```python
from build123d import *

# Parameters (mm, degrees)
BOSS_EXTRUDE1_DEPTH         = 6.35
FILLET1_R                   = 6.35
FILLET2_R                   = 1.5875
F_1_4_0_25_DIAMETER_HOLE1_D = 6.35


with BuildPart() as part:
    # Sketch2 → Boss-Extrude1 (new body)
    with BuildSketch(Plane.XY):
        with BuildLine():
            Line((-47.625, -279.4), (-26.924, -279.4))
            Line((-26.924, -279.4), (-26.924, -254))
            ThreePointArc((-26.924, -254), (0, -227.076), (26.924, -254))
            Line((26.924, -254), (26.924, -279.4))
            Line((26.924, -279.4), (47.625, -279.4))
            Line((47.625, -279.4), (47.625, 12.7))
            Line((47.625, 12.7), (26.924, 12.7))
            Line((26.924, 12.7), (26.924, -44.45))
            ThreePointArc((26.924, -44.45), (0, -71.374), (-26.924, -44.45))
            Line((-26.924, -44.45), (-26.924, 12.7))
            Line((-26.924, 12.7), (-47.625, 12.7))
            Line((-47.625, 12.7), (-47.625, -279.4))
        make_face()
    extrude(amount=BOSS_EXTRUDE1_DEPTH)

    # Fillet1
    fillet1_edges = [part.edges().sort_by_distance(p)[0] for p in [
        (-26.924, 12.7, 3.175),
        (26.924, 12.7, 3.175),
        (26.924, -279.4, 3.175),
        (-26.924, -279.4, 3.175),
    ]]
    fillet(fillet1_edges, radius=FILLET1_R)

    # Fillet2
    fillet2_edges = [part.edges().sort_by_distance(p)[0] for p in [
        (-47.625, 12.7, 3.175),
        (47.625, 12.7, 3.175),
        (47.625, -279.4, 3.175),
        (-47.625, -279.4, 3.175),
    ]]
    fillet(fillet2_edges, radius=FILLET2_R)

    # 1/4 (0.25) Diameter Hole1 (through all)
    with Locations(Plane.XY.offset(6.35)):
        with Locations((-25.4, -222.25), (-38.89375, -31.75), (38.89375, -31.75), (25.4, -222.25)):
            Hole(F_1_4_0_25_DIAMETER_HOLE1_D / 2)


solid = part.part
```
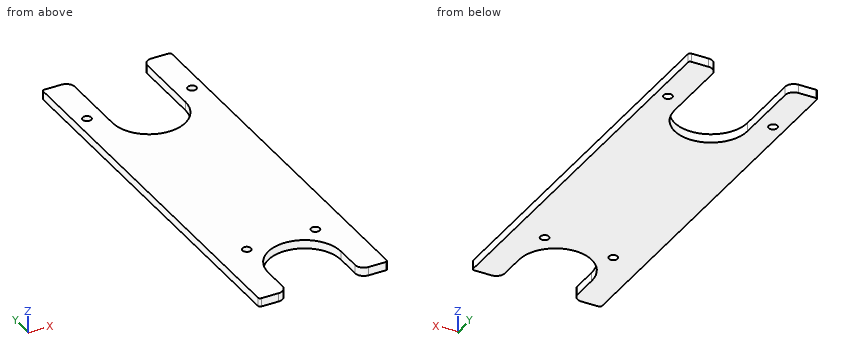
Part model, mm, in its own coordinate system. Round coordinates to 2 decimals unless told otherwise and drop trailing zeros. Loops run counter-clockwise (first coordinate to the right, second up) from the corner with the lowest first, then second, coordinate; pieces in that order, holes last.
Item 1: Cut at A-A, the plane y = -31.75. Give the cut face in (x, z) (3 decimals).
Item 2: Cut at B-B, the plane z = 3.5. State how many separate pieces and enclosed holes the cut face has, then the cut area to 3 significant figures.
Item 3: Cut at D-D, the plane x = 0. Give the cut face in (y, z), then the cut area to 3 significant figures.
Item 4: Drill centre lines: line 1 (X direction, y = -222.25, z = 3.25) (3 decimals); line 2 (X direction, y = -264.5, z = 5.5) (3 decimals); line 3 (X direction, y = -29, z = 1.5) (3 decimals). Where is each one in solid material? Low to high.
Item 5: Cut at C-C, the plane y = -222.25. Give the cut face in (x, z) (3 decimals).
Item 6: Drop a flat-ended pin along its axis: P1, Ø8.5, axis at x = -38.89, y = -31.75, coming from the -Z side. Give the stop position or say it passes through.
A:
1. outline: (-47.625, 0) - (-42.069, 0) - (-42.069, 6.35) - (-47.625, 6.35) - close; (-35.719, 0) - (-26.924, 0) - (-26.924, 6.35) - (-35.719, 6.35) - close; (26.924, 0) - (35.719, 0) - (35.719, 6.35) - (26.924, 6.35) - close; (42.069, 0) - (47.625, 0) - (47.625, 6.35) - (42.069, 6.35) - close
2. separate pieces: 1
2. enclosed holes: 4
2. area: 20,900 mm2
3. outline: (-227.08, 0) - (-71.37, 0) - (-71.37, 6.35) - (-227.08, 6.35) - close
3. area: 989 mm2
4. line 1: x = -47.625 to -28.575, -22.225 to 22.225, 28.575 to 47.625
4. line 2: x = -47.625 to -26.924, 26.924 to 47.625
4. line 3: x = -47.625 to -40.481, -37.307 to -26.924, 26.924 to 37.307, 40.481 to 47.625
5. outline: (-47.625, 0) - (-28.575, 0) - (-28.575, 6.35) - (-47.625, 6.35) - close; (-22.225, 0) - (22.225, 0) - (22.225, 6.35) - (-22.225, 6.35) - close; (28.575, 0) - (47.625, 0) - (47.625, 6.35) - (28.575, 6.35) - close
6. P1: stops at z = 0
